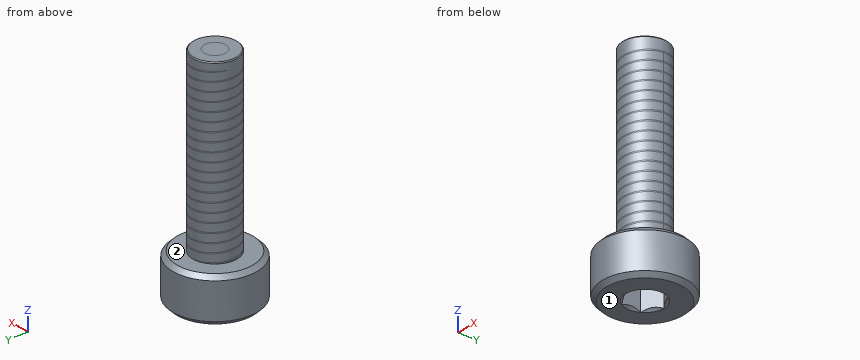
from build123d import *

# Parameters (mm, degrees)
SKETCH1_R            = 1
EXTRUDE1_DEPTH       = 8
CUT_SWEEP1_PITCH     = 0.4
SKETCH6_R            = 1.9
EXTRUDE2_DEPTH       = 2
CUT_EXTRUDE1_DEPTH   = 1.125
CHAMFER1_SIZE        = 0.19
SKETCH10_R           = 1
PARTIAL_THREAD_DEPTH = 8
CHAMFER2_SIZE        = 0.04


with BuildPart() as part:
    # Sketch1 → Extrude1 (new body)
    with BuildSketch(Plane.XY):
        Circle(SKETCH1_R)
    extrude(amount=-EXTRUDE1_DEPTH)

    # Cut-Sweep1: the profile of Sketch3 profile screwed along a right-hand helix of 21 turns, 6 arcs to a turn; built about Z, then put on its axis
    cut_sweep1_z = Axis((0, 0, 0), (0, 0, 1))
    cut_sweep1_corners = [(1.0003, 0, -0.350173205), (0.740192379, 0, -0.2), (0.740192379, 0, -0.15), (1.0003, 0, 0.000173205)]
    with BuildLine(mode=Mode.PRIVATE) as cut_sweep1_profile:
        Line(cut_sweep1_corners[0], cut_sweep1_corners[1])
        Line(cut_sweep1_corners[1], cut_sweep1_corners[2])
        Line(cut_sweep1_corners[2], cut_sweep1_corners[3])
        Line(cut_sweep1_corners[3], cut_sweep1_corners[0])
    cut_sweep1_cap = Face(cut_sweep1_profile.wire())
    cut_sweep1_turn_angles = [0, 30, 60, 90, 120, 150, 180, 210, 240, 270, 300, 330, 360]
    cut_sweep1_turn_weights = [1, 0.8660254037844387, 1, 0.8660254037844387, 1, 0.8660254037844387, 1, 0.8660254037844387, 1, 0.8660254037844387, 1, 0.8660254037844387, 1]
    cut_sweep1_turn_rails = [Edge.make_bspline([Vector(p[0], p[1], 0).rotate(cut_sweep1_z, cut_sweep1_turn_angles[k]) / cut_sweep1_turn_weights[k] + Vector(0, 0, p[2] + CUT_SWEEP1_PITCH * cut_sweep1_turn_angles[k] / 360) for k in range(13)], [0, 0, 0, 1, 1, 2, 2, 3, 3, 4, 4, 5, 5, 6, 6, 6], 2, cut_sweep1_turn_weights) for p in cut_sweep1_corners]
    cut_sweep1_turn_sides = [Face.make_surface_from_curves(cut_sweep1_turn_rails[p[0]], cut_sweep1_turn_rails[p[1]]) for p in [(0, 1), (1, 2), (2, 3), (3, 0)]]
    cut_sweep1 = Plane(origin=(0, 0, 0), x_dir=(0, 1, 0), z_dir=(0, 0, -1)) * Solid(Shell([*[p.moved(Location((0, 0, CUT_SWEEP1_PITCH * i))) for i in range(21) for p in cut_sweep1_turn_sides], cut_sweep1_cap, cut_sweep1_cap.rotate(cut_sweep1_z, 7560).moved(Location((0, 0, CUT_SWEEP1_PITCH * 7560 / 360)))]))
    add(cut_sweep1, mode=Mode.SUBTRACT)

    # Sketch4 → Cut-Revolve1 (revolve, cut)
    with BuildSketch(Plane(origin=(0, 0, 0), x_dir=(0, 0, -1), z_dir=(1, 0, 0)), mode=Mode.PRIVATE) as cut_revolve1_sk:
        Polygon((0.35977197, 1), (0, 0.486192379), (0, 1), align=None)
    revolve(cut_revolve1_sk.sketch.rotate(Axis((0, 0, 0), (0, 0, -1)), 278.428757719), axis=Axis((0, 0, 0), (0, 0, -1)), mode=Mode.SUBTRACT)

    # Sketch6 → Extrude2 (add)
    with BuildSketch(Plane(origin=(0, 0, -8), x_dir=(-1, 0, 0), z_dir=(0, 0, -1))):
        Circle(SKETCH6_R)
    extrude(amount=EXTRUDE2_DEPTH)

    # Sketch7 → Cut-Extrude1 (cut)
    with BuildSketch(Plane(origin=(0, 0, -10), x_dir=(-1, 0, 0), z_dir=(0, 0, -1))):
        Polygon((0, 0.866025404), (-0.75, 0.433012702), (-0.75, -0.433012702), (0, -0.866025404), (0.75, -0.433012702), (0.75, 0.433012702), align=None)
    extrude(amount=-CUT_EXTRUDE1_DEPTH, mode=Mode.SUBTRACT)

    # Cut-Extrude2 cone 1 section (through the dimple's axis) → Cut-Extrude2 (revolve, cut)
    with BuildSketch(Plane(origin=(0, 0, -10), x_dir=(0, 1, 0), z_dir=(1, 0, 0))):
        Polygon((0, 0), (0.866025404, 0), (0, 0.866025404), align=None)
    revolve(axis=Axis((0, 0, -10), (0, 0, 1)), mode=Mode.SUBTRACT)

    # Chamfer1
    chamfer1_edges = [part.edges().sort_by_distance(p)[0] for p in [
        (1.9, 0, -8),
        (1.9, 0, -10),
    ]]
    chamfer(chamfer1_edges, length=CHAMFER1_SIZE)


with BuildPart() as body_2:
    # Sketch10 → partial thread (new body)
    with BuildSketch(Plane.XY.offset(-8)):
        Circle(SKETCH10_R)
    extrude(amount=PARTIAL_THREAD_DEPTH)

    # Chamfer2
    chamfer2_edges = [body_2.edges().sort_by_distance(p)[0] for p in [
        (-1, 0, 0),
    ]]
    chamfer(chamfer2_edges, length=CHAMFER2_SIZE)


with BuildPart() as part_1:
    add(part.part)

    # Combine1: union body 2
    add(body_2.part)


solid = part_1.part
The model under review builds one solid part; all positions refer to its coordinate system, in mm. Face numbers are marked on the shaded views. A direction names the side the tool comes from. Give positions to 0.01 mm unless a question says otherwise; leave off trailing zeros. Order: outer loops, then holes, each group sorted by start corner. A loop starts at its lowest first (then second) coordinate and runs counter-clockwise, first axis right, second up. Notation, with made-up numbers: M -38,-21.75 L -2,-21.75 A22 cw -2,7.25 Z; hole C -31,38 d11. An arc over 180 degrees is marked long. Answer in a Markdown table with one row per item. Add a question column.
1. Machinability: for the marked faces 1 and 2, which of the approach directions +Z, -Z, +X, -X, +Y, -Y give a long, thin tool a straight path to every point of the face, cutting with its end or side? Answer none if there is none.
2. For pin 1 Ø0.8 at (x, y) = (0, 0) entering from -Z (3 decimals), flat-tipped, find the tip position at first contact; note if it passes through.
3. To check wall thickness, follow line 1 along Z through (x, y) = (1.45, 0.6); line 2 along Y through (x, z) = (0.9, -1.5); line 3 along Y through (x, z) = (0.3, -1.25). State the ranges of each line that lie inside material, in increasing order.
4. Add section A-A on z = -1.5. State the section outline as (x, y) points.
The answers:
| question | item | result |
|---|---|---|
| 1 | face 1 | -Z, +X, -X, +Y, -Y |
| 1 | face 2 | +Z |
| 2 | pin 1 | z = -8.875 |
| 3 | line 1 | -10 to -8 |
| 3 | line 2 | -0.44 to 0.44 |
| 3 | line 3 | -0.95 to 0.95 |
| 4 | outline | C 0,0 d2 |
